Source: CAD feature listing. Evaluate the final solid. Frame: model axes, mm. A direction names the side the tool comes from. Give positions to 0.01 mm unless a question says otherwise; leave off trailing zeros. Write each loop counter-clockwise with the first axis right and the second up, starting at its lowest first coordinate (ties: lowest second). Pieces come first, ordered by that corner, then holes. Notation, with made-up numbers: M -23,-36 L -11,-36 A21 cw -11,-6 Z; hole C 21,33.25 d11. An arc over 180 degrees is marked long. Answer as a JSON object with one key per item and string values. Group by question number.
```python
from build123d import *

# Parameters (mm, degrees)
SKETCH_1_W                   = 100
SKETCH_1_H                   = 24
EXTRUDE_1_DEPTH              = 13.3
SKETCH_2_W                   = 90
SKETCH_2_H                   = 24
CUT_EXTRUDE_1_DEPTH          = 9.3
HOLE_WIZARD_3_2_3_2_1_D      = 3.2
SKETCH_5_R                   = 5
CUT_EXTRUDE_2_DEPTH          = 53.254090749
SKETCH_6_R                   = 6
CUT_EXTRUDE_3_DEPTH          = 0.5
HOLE_WIZARD_M2_1_D           = 2.4
HOLE_WIZARD_M2_1_CBORE_D     = 6
HOLE_WIZARD_M2_1_CBORE_DEPTH = 2
PATTERN_CIRCULAR_1_COUNT     = 3
SKETCH_9_R                   = 1.1
CUT_EXTRUDE_4_DEPTH          = 10


with BuildPart() as part:
    # 草图1 → 凸台-拉伸1 (new body)
    with BuildSketch(Plane(origin=(0, 0, 0), x_dir=(1, 0, 0), z_dir=(0, 1, 0))):
        Rectangle(SKETCH_1_W, SKETCH_1_H)
    extrude(amount=EXTRUDE_1_DEPTH)

    # 草图2 → 切除-拉伸1 (cut)
    with BuildSketch(Plane(origin=(0, 13.3, 0), x_dir=(1, 0, 0), z_dir=(0, 1, 0))):
        Rectangle(SKETCH_2_W, SKETCH_2_H)
    extrude(amount=-CUT_EXTRUDE_1_DEPTH, mode=Mode.SUBTRACT)

    # Ø3.2 (3.2) 直径孔1 (through all)
    with Locations(Plane(origin=(50, 0, 0), x_dir=(0, 0, -1), z_dir=(1, 0, 0))):
        with Locations((8.5, 8.8), (-8.5, 8.8)):
            Hole(HOLE_WIZARD_3_2_3_2_1_D / 2)

    # 草图5 → 切除-拉伸2 (cut, through all)
    with BuildSketch(Plane(origin=(0, 4, 0), x_dir=(1, 0, 0), z_dir=(0, 1, 0))):
        with Locations(Location((0, 0, 0), (0, 0, 270))):
            Circle(SKETCH_5_R)
    extrude(amount=-CUT_EXTRUDE_2_DEPTH, mode=Mode.SUBTRACT)

    # 草图6 → 切除-拉伸3 (cut)
    with BuildSketch(Plane(origin=(0, 4, 0), x_dir=(1, 0, 0), z_dir=(0, 1, 0))):
        with Locations(Location((0, 0, 0), (0, 0, 270))):
            Circle(SKETCH_6_R)
    extrude(amount=-CUT_EXTRUDE_3_DEPTH, mode=Mode.SUBTRACT)

    # M2 六角头螺栓的柱形沉头孔1 (through all)
    with Locations(Plane(origin=(0, 4, 0), x_dir=(1, 0, 0), z_dir=(0, 1, 0))):
        with Locations((9.5, 0)):
            hole_wizard_m2_1 = CounterBoreHole(HOLE_WIZARD_M2_1_D / 2, HOLE_WIZARD_M2_1_CBORE_D / 2, HOLE_WIZARD_M2_1_CBORE_DEPTH)

    # 阵列(圆周)1: M2 六角头螺栓的柱形沉头孔1 ×3 about axis
    pattern_circular_1_axis = Axis((0, 0, 0), (0, 1, 0))
    for i in range(1, PATTERN_CIRCULAR_1_COUNT):
        add(hole_wizard_m2_1.rotate(pattern_circular_1_axis, i * 360 / PATTERN_CIRCULAR_1_COUNT), mode=Mode.SUBTRACT)

    # 草图9 → 切除-拉伸4 (cut)
    with BuildSketch(Plane.XY.offset(12)):
        with Locations((0, 1.5)):
            Circle(SKETCH_9_R)
    extrude(amount=-CUT_EXTRUDE_4_DEPTH, mode=Mode.SUBTRACT)


solid = part.part
```
(1) Access query for faces 4 (the flat face through (-3.9, 2, -9.4)), 5 (the cylindrical face through (47.47, 9.88, 7.32)), 6 (the cylindrical face through (0.59, 2.43, 8.49)), 7 (the flat face through (-45, 9, 0)). Directions: +Z, -Z, +X, -X, +Y, -Y. A direction counts if a zero-diameter tool reaches every point of the face in a straight line with its end or side. Return the directions, or none.
(2) Section A-A, the plane x = 0. Return loops of the section in (y, z).
(3) Contact query for flat-ended pins moving along their axis: pin 1 Ø9.5 at (x, z) = (-2, -0.5) entering from +Y; pin 2 Ø1.8 at (x, z) = (9, -1) entering from +Y. Output: stop coordinate, or through.
(4) Section C-C, the plane y = 8.8. Return loops of the section in (x, z).
(5) Section B-B, the plane z = 0. Return loops of the section in (x, y), plus the area to 3 significant figures.
(6) Section D-D, the plane z = 8.5. Return loops of the section in (x, y).
(7) Pull-direction query (Z, two-part tool) for faces 1 (the cylindrical face through (12.27, 3.01, 1.15)), 2 (the flat face through (-50, 7, 0)), 3 (the flat face through (-11.8, 3.6, 12)); classes: pulls with the +Z half, pulls with the -Z half, needs draft (parallel to the pull), parting line crosses it, or undercut.
(8) Ray query, L1, parallel to X at y = 11.25, z = 5.75; L2, parallel to Y at x = 4.5, z = -9; L3, parallel to Y at x = 0, z = 8.75. Return the intervals inside material, ascending. Write a range as [from, to].
Reported:
{
 "1": {"face 4": "+Y", "face 5": "+X, -X", "face 6": "+Z", "face 7": "+Z, -Z, +Y"},
 "2": {"outline": "M 0,-12 L 4,-12 L 4,-6 L 3.5,-6 L 3.5,-5 L 0,-5 Z; M 0,5 L 0.4,5 L 0.4,12 L 0,12 Z; M 2.6,5 L 3.5,5 L 3.5,6 L 4,6 L 4,12 L 2.6,12 Z"},
 "3": {"pin 1": "stops at y = 4", "pin 2": "stops at y = 2"},
 "4": {"outline": "M -50,-12 L -45,-12 L -45,-10.1 L -50,-10.1 Z; M -50,-6.9 L -45,-6.9 L -45,6.9 L -50,6.9 Z; M -50,10.1 L -45,10.1 L -45,12 L -50,12 Z; M 45,-12 L 50,-12 L 50,-10.1 L 45,-10.1 Z; M 45,-6.9 L 50,-6.9 L 50,6.9 L 45,6.9 Z; M 45,10.1 L 50,10.1 L 50,12 L 45,12 Z"},
 "5": {"outline": "M -50,0 L -5,0 L -5,3.5 L -6,3.5 L -6,4 L -45,4 L -45,13.3 L -50,13.3 Z; M 5,0 L 8.3,0 L 8.3,2 L 6.5,2 L 6.5,4 L 6,4 L 6,3.5 L 5,3.5 Z; M 10.7,0 L 50,0 L 50,13.3 L 45,13.3 L 45,4 L 12.5,4 L 12.5,2 L 10.7,2 Z", "area": "435 mm2"},
 "6": {"outline": "M -50,0 L -5.92,0 L -5.92,2 L -7.74,2 L -7.74,4 L -45,4 L -45,7.2 L -50,7.2 Z; M -50,10.4 L -45,10.4 L -45,13.3 L -50,13.3 Z; M -3.58,0 L 50,0 L 50,7.2 L 45,7.2 L 45,4 L -1.76,4 L -1.76,2 L -3.58,2 Z; M 45,10.4 L 50,10.4 L 50,13.3 L 45,13.3 Z; hole C 0,1.5 d2.2"},
 "7": {"face 1": "undercut", "face 2": "needs draft", "face 3": "pulls with the +Z half"},
 "8": {"L1": "x = [-50, -45], [45, 50]", "L2": "y = [0, 4]", "L3": "y = [0, 0.4], [2.6, 4]"}
}
